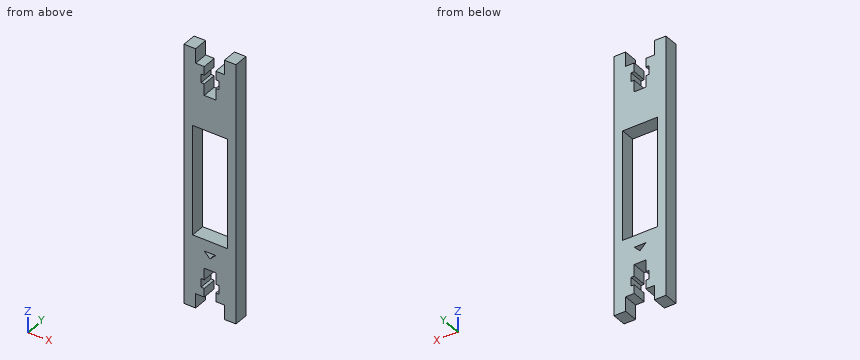
```python
from build123d import *

# Parameters (mm, degrees)
SKETCH1_W           = 12
SKETCH1_H           = 38
BOSS_EXTRUDE4_DEPTH = 5


with BuildPart() as part:
    # Sketch1 → Boss-Extrude4 (new body)
    with BuildSketch(Plane(origin=(0, 0, 0), x_dir=(1, 0, 0), z_dir=(0, 1, 0))):
        Polygon((-8.645320197, 61.366995074), (-5.645320197, 61.366995074), (-5.645320197, 58.366995074), (-6.745320197, 58.366995074), (-6.745320197, 55.366995074), (-5.645320197, 55.366995074), (-5.645320197, 51.366995074), (-1.645320197, 51.366995074), (-1.645320197, 55.366995074), (-0.545320197, 55.366995074), (-0.545320197, 58.366995074), (-1.645320197, 58.366995074), (-1.645320197, 61.366995074), (1.354679803, 61.366995074), (1.354679803, 66.366995074), (5.354679803, 66.366995074), (5.354679803, 61.366995074), (5.354679803, 16.366995074), (5.354679803, -3.633004926), (5.354679803, -18.633004926), (5.354679803, -23.633004926), (1.354679803, -23.633004926), (1.354679803, -18.633004926), (-1.645320197, -18.633004926), (-1.645320197, -15.633004926), (-0.545320197, -15.633004926), (-0.545320197, -12.633004926), (-1.645320197, -12.633004926), (-1.645320197, -8.633004926), (-5.645320197, -8.633004926), (-5.645320197, -12.633004926), (-6.745320197, -12.633004926), (-6.745320197, -15.633004926), (-5.645320197, -15.633004926), (-5.645320197, -18.633004926), (-8.645320197, -18.633004926), (-8.645320197, -23.633004926), (-12.645320197, -23.633004926), (-12.645320197, -18.633004926), (-12.645320197, -3.633004926), (-12.645320197, 16.366995074), (-12.645320197, 61.366995074), (-12.645320197, 66.366995074), (-8.645320197, 66.366995074), align=None)
        with Locations((-3.645320197, 22.366995074)):
            Rectangle(SKETCH1_W, SKETCH1_H, mode=Mode.SUBTRACT)
        Polygon((-5.645320197, 45.366995074), (-1.645320197, 45.366995074), (-3.645320197, 47.366995074), align=None, mode=Mode.SUBTRACT)
    extrude(amount=BOSS_EXTRUDE4_DEPTH)


solid = part.part
```
Can you work these out from the model? Positions are in its coordinate system, mm. Coordinates: 2 decimals unless noted, no trailing zeros. Write each loop counter-clockwise with the first axis right and the second up, starting at its lowest first coordinate (ties: lowest second). Pieces come first, ordered by that corner, then holes. Notation, with made-up numbers: (40.25, 35.5) - (49.25, 35.5) arc R17 cw to (49.25, 57.5) - close; hole circle Ø2 at (-9.5, 30). An arc over 180 degrees is marked (long way). Return JSON: item names as keys, results as strings.
Q1. If we section it at C-C (y = 3.25): Count the separate pieces of the cut face and the enclosed holes in it, then the cut area to 3 significant figures.
Computed values:
{"separate pieces": "1", "enclosed holes": "2", "area": "967 mm2"}
Q2. Please list where these lines run through material, in increasing order: L1, parallel to Z at x = -6.5, y = 4.1; L2, parallel to X at y = 4.3, z = 17.5; L3, parallel to X at y = 0.45, z = -11. Write a range as from..to.
Computed values:
{"L1": "z = -61.37..-58.37, -55.37..-41.37, -3.37..12.63, 15.63..18.63", "L2": "x = -12.65..-5.65, -1.65..5.35", "L3": "x = -12.65..-9.65, 2.35..5.35"}
Q3. If we section it at B-B (x = -2.75): Please give me the cut outline in (y, z), then the cut area to 3 significant figures.
Computed values:
{"outline": "(0, -51.37) - (5, -51.37) - (5, -46.47) - (0, -46.47) - close; (0, -45.37) - (5, -45.37) - (5, -41.37) - (0, -41.37) - close; (0, -3.37) - (5, -3.37) - (5, 8.63) - (0, 8.63) - close", "area": "104 mm2"}
Q4. If we section it at A-A (z = -35): Please give me the cut outline in (x, y), then the cut area to 3 significant figures.
Computed values:
{"outline": "(-12.65, 0) - (-9.65, 0) - (-9.65, 5) - (-12.65, 5) - close; (2.35, 0) - (5.35, 0) - (5.35, 5) - (2.35, 5) - close", "area": "30.0 mm2"}
Q5. I'm going to push flat-ended pins straight in: pin 1 Ø0.6 at (x, y) = (-1, 2) entering from +Z; pin 2 Ø0.6 at (x, y) = (-1, 3) entering from -Z; pin 3 Ø1.2 at (x, y) = (-4.5, 1.5) entering from -Z. Where does each tip first touch, or does it pass through?
Computed values:
{"pin 1": "stops at z = 18.63", "pin 2": "stops at z = -61.37", "pin 3": "stops at z = -51.37"}
Q6. If we section it at D-D (z = 14): Please give me the cut outline in (x, y).
Computed values:
{"outline": "(-12.65, 0) - (-6.75, 0) - (-6.75, 5) - (-12.65, 5) - close; (-0.55, 0) - (5.35, 0) - (5.35, 5) - (-0.55, 5) - close"}
